CAD build for the part. Positions are in the model's coordinates, mm. Face numbers are marked on the shaded views. Coordinates: 2 decimals unless noted, no trailing zeros. Write each loop counter-clockwise with the first axis right and the second up, starting at its lowest first coordinate (ties: lowest second). Pieces come first, ordered by that corner, then holes.
```python
from build123d import *

# Parameters (mm, degrees)
F0_R     = 1.5875
F1_DEPTH = 25.4


with BuildPart() as f1:
    # F0 (on Front) → F1 (new body)
    with BuildSketch(Plane.XZ):
        with BuildLine():
            ThreePointArc((-53.4077063203, 56.5580051482), (-46.6725142295, 59.3478130574), (-43.8827063203, 66.0830051482))
            ThreePointArc((-43.8827063203, 66.0830051482), (-53.4077063203, 75.6080051482), (-62.9327063203, 66.0830051482))
            ThreePointArc((-62.9327063203, 66.0830051482), (-60.1428984111, 59.3478130574), (-53.4077063203, 56.5580051482))
        make_face()
        with BuildLine():
            ThreePointArc((-50.2327063203, 66.0830051482), (-51.16264229, 63.8379411179), (-53.4077063203, 62.9080051482))
            ThreePointArc((-53.4077063203, 62.9080051482), (-55.6527703506, 68.3280691784), (-50.2327063203, 66.0830051482))
        make_face(mode=Mode.SUBTRACT)
        with BuildLine():
            Line((-37.6602494156, 17.2912944785), (-43.8827063203, 66.0830051482))
            ThreePointArc((-43.8827063203, 66.0830051482), (-46.6725142295, 59.3478130574), (-53.4077063203, 56.5580051482))
            Line((-53.4077063203, 56.5580051482), (-53.4077063203, 31.1580051482))
            ThreePointArc((-53.4077063203, 31.1580051482), (-42.9164234654, 27.1972239249), (-37.6602494156, 17.2912944785))
        make_face()
        with BuildLine():
            ThreePointArc((-53.4077063203, 56.5580051482), (-60.1428984111, 59.3478130574), (-62.9327063203, 66.0830051482))
            Line((-62.9327063203, 66.0830051482), (-69.155163225, 17.2912944785))
            ThreePointArc((-69.155163225, 17.2912944785), (-63.8989891751, 27.1972239249), (-53.4077063203, 31.1580051482))
            Line((-53.4077063203, 31.1580051482), (-53.4077063203, 56.5580051482))
        make_face()
        with Locations((-58.4421381354, 52.9512051482)):
            Circle(F0_R, mode=Mode.SUBTRACT)
        with BuildLine():
            ThreePointArc((-37.5327063203, 15.2830051482), (-37.5646241807, 16.2891727877), (-37.6602494156, 17.2912944785))
            ThreePointArc((-37.6602494156, 17.2912944785), (-42.9164234654, 27.1972239249), (-53.4077063203, 31.1580051482))
            Line((-53.4077063203, 31.1580051482), (-53.4077063203, 18.4580051482))
            ThreePointArc((-53.4077063203, 18.4580051482), (-51.16264229, 17.5280691784), (-50.2327063203, 15.2830051482))
            ThreePointArc((-50.2327063203, 15.2830051482), (-51.16264229, 13.0379411179), (-53.4077063203, 12.1080051482))
            Line((-53.4077063203, 12.1080051482), (-53.4077063203, -0.5919948518))
            ThreePointArc((-53.4077063203, -0.5919948518), (-42.9164234654, 3.3687863714), (-37.6602494156, 13.2747158178))
            ThreePointArc((-37.6602494156, 13.2747158178), (-37.5646241807, 14.2768375086), (-37.5327063203, 15.2830051482))
        make_face()
        with BuildLine():
            ThreePointArc((-53.4077063203, 31.1580051482), (-63.8989891751, 27.1972239249), (-69.155163225, 17.2912944785))
            ThreePointArc((-69.155163225, 17.2912944785), (-69.2827063203, 15.2830051482), (-69.155163225, 13.2747158178))
            ThreePointArc((-69.155163225, 13.2747158178), (-63.8989891751, 3.3687863714), (-53.4077063203, -0.5919948518))
            Line((-53.4077063203, -0.5919948518), (-53.4077063203, 12.1080051482))
            ThreePointArc((-53.4077063203, 12.1080051482), (-56.5827063203, 15.2830051482), (-53.4077063203, 18.4580051482))
            Line((-53.4077063203, 18.4580051482), (-53.4077063203, 31.1580051482))
        make_face()
        with BuildLine():
            ThreePointArc((-53.4077063203, -0.5919948518), (-63.8989891751, 3.3687863714), (-69.155163225, 13.2747158178))
            Line((-69.155163225, 13.2747158178), (-62.9327063203, -48.2169948518))
            ThreePointArc((-62.9327063203, -48.2169948518), (-60.1428984111, -41.481802761), (-53.4077063203, -38.6919948518))
            Line((-53.4077063203, -38.6919948518), (-53.4077063203, -0.5919948518))
        make_face()
        with BuildLine():
            Line((-42.102295446, -30.6225764362), (-37.6602494156, 13.2747158178))
            ThreePointArc((-37.6602494156, 13.2747158178), (-42.9164234654, 3.3687863714), (-53.4077063203, -0.5919948518))
            Line((-53.4077063203, -0.5919948518), (-53.4077063203, -38.6919948518))
            ThreePointArc((-53.4077063203, -38.6919948518), (-46.6725142295, -41.481802761), (-43.8827063203, -48.2169948518))
            Line((-43.8827063203, -48.2169948518), (-16.8952063203, -48.2169948518))
            ThreePointArc((-16.8952063203, -48.2169948518), (-14.570366396, -42.6043347762), (-8.9577063203, -40.2794948518))
            Line((-8.9577063203, -40.2794948518), (-34.4762444457, -39.3681184902))
            ThreePointArc((-34.4762444457, -39.3681184902), (-40.1845456585, -36.6480145197), (-42.102295446, -30.6225764362))
        make_face()
        with BuildLine():
            ThreePointArc((-53.4077063203, -38.6919948518), (-60.1428984111, -41.481802761), (-62.9327063203, -48.2169948518))
            ThreePointArc((-62.9327063203, -48.2169948518), (-60.1953592391, -54.8993142736), (-53.556665826, -57.7408300071))
            Line((-53.556665826, -57.7408300071), (-52.5845948483, -57.7063632452))
            ThreePointArc((-52.5845948483, -57.7063632452), (-46.3875296213, -54.6545987628), (-43.8827063203, -48.2169948518))
            Line((-43.8827063203, -48.2169948518), (-50.2327063203, -48.2169948518))
            ThreePointArc((-50.2327063203, -48.2169948518), (-55.6527703506, -50.4620588821), (-53.4077063203, -45.0419948518))
            Line((-53.4077063203, -45.0419948518), (-53.4077063203, -38.6919948518))
        make_face()
        with BuildLine():
            Line((-52.5845948483, -57.7063632452), (-53.556665826, -57.7408300071))
            ThreePointArc((-53.556665826, -57.7408300071), (-53.0701900869, -57.7360130676), (-52.5845948483, -57.7063632452))
        make_face()
        with BuildLine():
            Line((-16.8952063203, -48.2169948518), (-43.8827063203, -48.2169948518))
            ThreePointArc((-43.8827063203, -48.2169948518), (-46.3875296213, -54.6545987628), (-52.5845948483, -57.7063632452))
            Line((-52.5845948483, -57.7063632452), (-8.6764427924, -56.1495100316))
            ThreePointArc((-8.6764427924, -56.1495100316), (-14.4700278366, -53.9282309484), (-16.8952063203, -48.2169948518))
        make_face()
        with BuildLine():
            ThreePointArc((-1.0202063203, -48.2169948518), (-3.3450462446, -42.6043347762), (-8.9577063203, -40.2794948518))
            ThreePointArc((-8.9577063203, -40.2794948518), (-14.570366396, -42.6043347762), (-16.8952063203, -48.2169948518))
            ThreePointArc((-16.8952063203, -48.2169948518), (-14.4700278366, -53.9282309484), (-8.6764427924, -56.1495100316))
            ThreePointArc((-8.6764427924, -56.1495100316), (-3.2464702237, -53.7293163681), (-1.0202063203, -48.2169948518))
        make_face()
        with BuildLine():
            ThreePointArc((-5.7827063203, -48.2169948518), (-8.9577063203, -51.3919948518), (-12.1327063203, -48.2169948518))
            ThreePointArc((-12.1327063203, -48.2169948518), (-8.9577063203, -45.0419948518), (-5.7827063203, -48.2169948518))
        make_face(mode=Mode.SUBTRACT)
        with BuildLine():
            ThreePointArc((-43.8827063203, -48.2169948518), (-46.6725142295, -41.481802761), (-53.4077063203, -38.6919948518))
            Line((-53.4077063203, -38.6919948518), (-53.4077063203, -45.0419948518))
            ThreePointArc((-53.4077063203, -45.0419948518), (-51.16264229, -45.9719308216), (-50.2327063203, -48.2169948518))
            Line((-50.2327063203, -48.2169948518), (-43.8827063203, -48.2169948518))
        make_face()
    extrude(amount=F1_DEPTH)


solid = f1.part
```
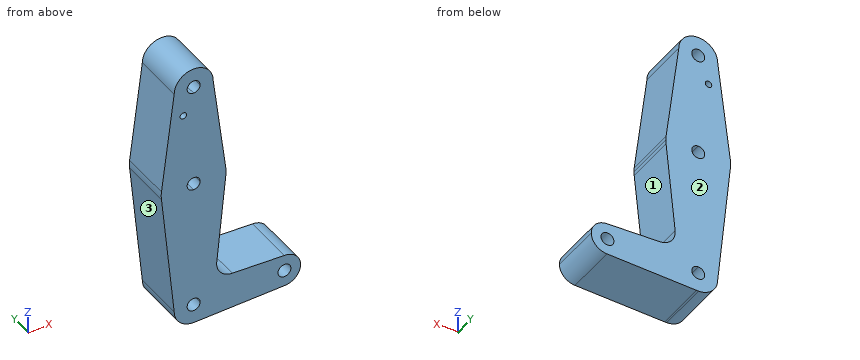
Item 1: Saw through at C-C, the plane z = -3. Write the cut outline in (x, y), and give its area (3 significant figures).
Item 2: Saw through at A-A, the plane y = -19.5. State how many separate pieces and enclosed holes the cut face has, and give its area (3 significant figures).
Item 3: Wall check: line 1 along X through (y, z) = (-14, -48); line 2 along X through (y, z) = (-1.5, 15); line 3 along Z through (x, y) = (-54, -7.75). Give the ranges that are in metal, low to high.
Item 4: Two-plate mould, pull along Z, no slides. Class the marked faces 1, 2 and 3: +Z half, -Z half, draft (parallel to the pull), parting line (faces both ways), or undercut.
Item 5: Saw through at D-D, the plane x = -21. Write the cut outline in (y, z), and give its area (3 significant figures).
Item 6: Flat gauge pins, fed straight in: pin 1 Ø12 at (x, y) = (-14.5, -6) entering from +Z; pin 2 Ø6 at (x, y) = (-13.5, -15) entering from -Z; pin 3 Ø4 at (y, z) = (-18.5, -24.5) entering from +X. Where does each tip first touch, or does it go through?
Item 7: Saw through at B-B, the plane z = 64.5. Write the cut outline in (x, y), and give its area (3 significant figures).
Working result:
1. outline: (-67.51, -25.4) - (-39.31, -25.4) - (-39.31, 0) - (-67.51, 0) - close
1. area: 716 mm2
2. separate pieces: 1
2. enclosed holes: 5
2. area: 3,790 mm2
3. line 1: x = -62.95 to -56.58, -50.24 to -12.13, -5.79 to -1.02
3. line 2: x = -69.28 to -56.57, -50.25 to -37.54
3. line 3: z = -57.72 to -51.34, -45.1 to 12.16, 18.4 to 62.96, 69.2 to 75.59
4. face 1: undercut
4. face 2: draft
4. face 3: -Z half
5. outline: (-25.4, -56.59) - (0, -56.59) - (0, -39.85) - (-25.4, -39.85) - close
5. area: 425 mm2
6. pin 1: stops at z = -39.87
6. pin 2: stops at z = -56.43
6. pin 3: stops at x = -41.28
7. outline: (-63.13, -25.4) - (-56.16, -25.4) - (-56.16, 0) - (-63.13, 0) - close; (-50.66, -25.4) - (-43.68, -25.4) - (-43.68, 0) - (-50.66, 0) - close
7. area: 354 mm2
